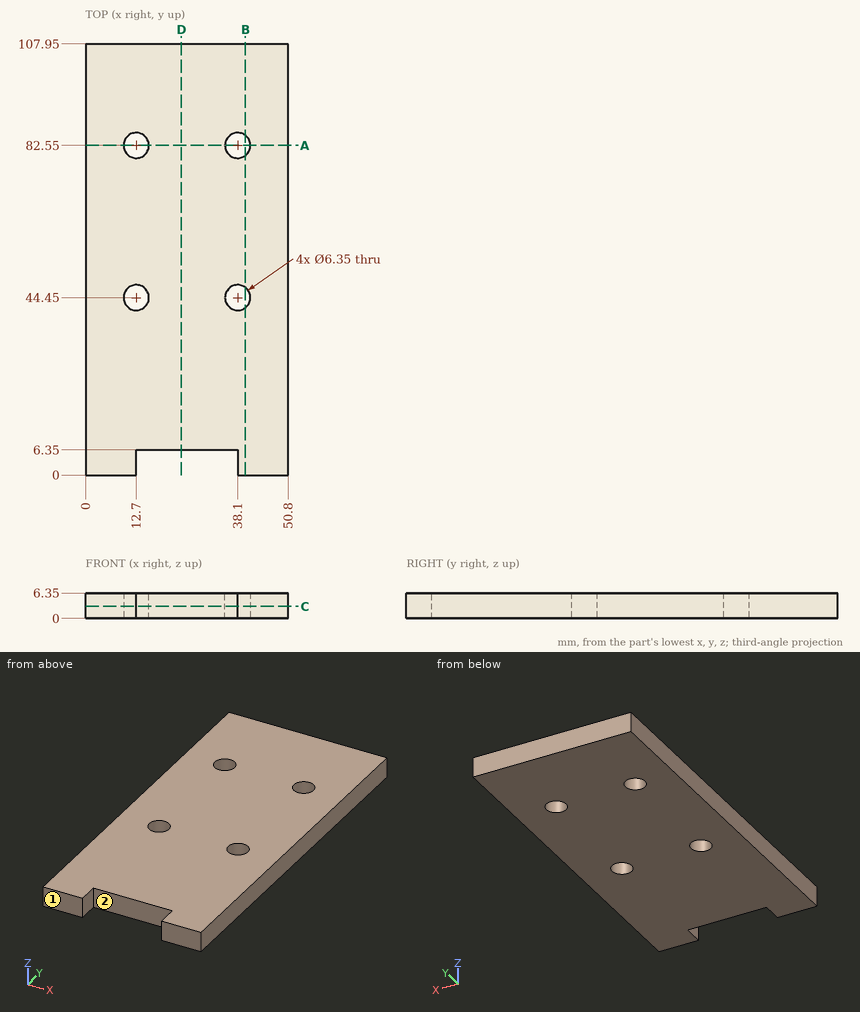
The figure shows three views and two pictorial views of one solid part (mm, origin at its lowest corner). Answer the questions. Coordinates: 2 decimals unless noted, no trailing zeros. Loops run counter-clockwise (first coordinate to the right, second up) from the corner with the lowest first, then second, coordinate; pieces in that order, holes last.
(1) The part is cut by section D-D (x = 24). Determine the outline of the cut face in (y, z), and give its area (3 significant figures).
Solution:
outline: (6.35, 0) - (107.95, 0) - (107.95, 6.35) - (6.35, 6.35) - close
area: 645 mm2
(2) Consider line 1 along Y through (x, z) = (38, 2.5); line 2 along X through (y, z) = (44.5, 5.75); line 3 along Y through (x, z) = (15.5, 1.5). Determine where each line is inside the solid, lowest interval first.
Solution:
line 1: y = 6.35 to 41.28, 47.62 to 79.38, 85.72 to 107.95
line 2: x = 0 to 9.53, 15.87 to 34.93, 41.27 to 50.8
line 3: y = 6.35 to 42.95, 45.95 to 81.05, 84.05 to 107.95
(3) The part is cut by section A-A (y = 82.55). Determine the outline of the cut face in (x, z) (3 decimals), and give its area (3 significant figures).
Solution:
outline: (0, 0) - (9.525, 0) - (9.525, 6.35) - (0, 6.35) - close; (15.875, 0) - (34.925, 0) - (34.925, 6.35) - (15.875, 6.35) - close; (41.275, 0) - (50.8, 0) - (50.8, 6.35) - (41.275, 6.35) - close
area: 242 mm2
(4) A flat-ended cylindrical pin translates along its axis: pin 1 Ø5.5 at (x, y) = (12.7, 82.55) entering from +Z. Find the tip coordinate at first contact, or state that the pin passes through.
Solution:
pin 1: passes through
(5) The part is cut by section C-C (z = 3). Determine the outline of the cut face in (x, y) (3 decimals), and give its area (3 significant figures).
Solution:
outline: (0, 0) - (12.7, 0) - (12.7, 6.35) - (38.1, 6.35) - (38.1, 0) - (50.8, 0) - (50.8, 107.95) - (0, 107.95) - close; hole circle Ø6.35 at (12.7, 44.45); hole circle Ø6.35 at (12.7, 82.55); hole circle Ø6.35 at (38.1, 44.45); hole circle Ø6.35 at (38.1, 82.55)
area: 5,200 mm2
(6) The part is cut by section B-B (x = 40). Determine the outline of the cut face in (y, z), and give its area (3 significant figures).
Solution:
outline: (0, 0) - (41.91, 0) - (41.91, 6.35) - (0, 6.35) - close; (46.99, 0) - (80.01, 0) - (80.01, 6.35) - (46.99, 6.35) - close; (85.09, 0) - (107.95, 0) - (107.95, 6.35) - (85.09, 6.35) - close
area: 621 mm2
(7) The mould has two halves that part along X. Classify the marked faces 1 and 2: released by +X, released by -X, zero draft, split by the parting line, or undercut.
Solution:
face 1: zero draft
face 2: undercut
